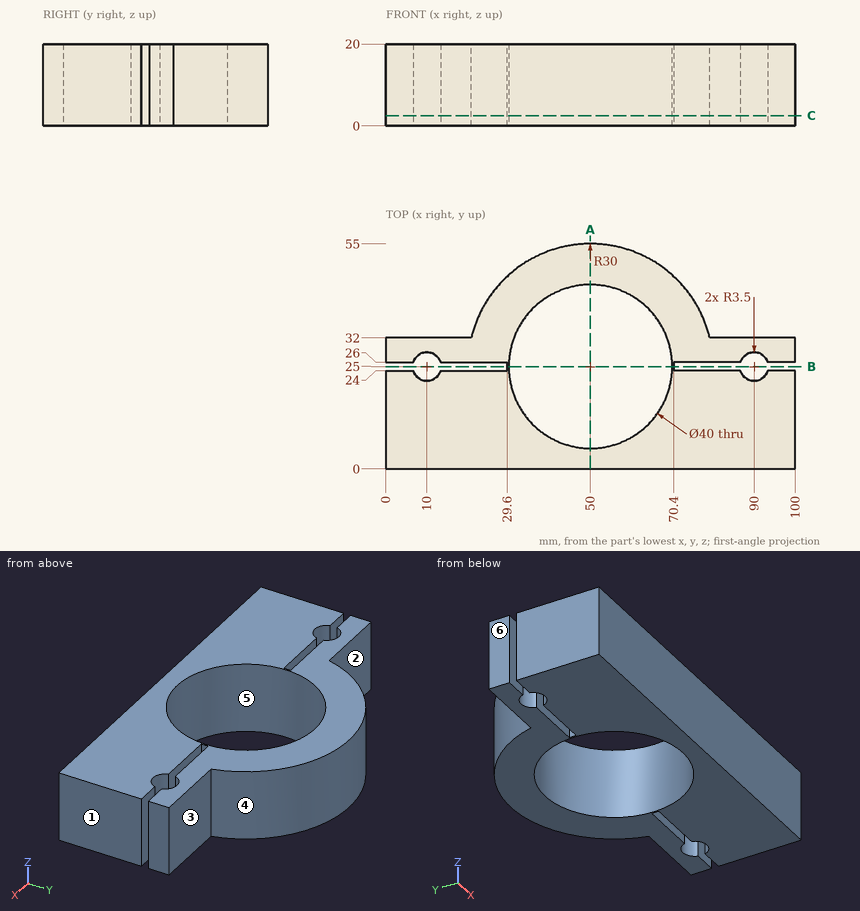
Geometry check sheet. Reference: drawing and pictorial views, mm from the part's lowest x, y, z. A direction names the side the tool comes from. Round coordinates to 2 decimals unless told otherwise and drop trailing zeros. Order: outer loops, then holes, each group sorted by start corner. A loop starts at its lowest first (then second) coordinate and runs counter-clockwise, first axis right, second up. Notation, with made-up numbers: M 62,43 L 118,43 A24 ccw 118,77 Z; hole C 75,-35.5 d10. An arc over 180 degrees is marked long. Write item = value, one per line.
Q1. Section check A-A (x = 50). Enter the section's corners in (y, z).
Answer block:
outline = M 0,0 L 5,0 L 5,20 L 0,20 Z; M 45,0 L 55,0 L 55,20 L 45,20 Z
Q2. Release check for a two-part mould opening along X. For the marked faces 4, 5 and 6 record: released by +X, released by -X, zero draft, split by the parting line, or undercut.
Answer block:
face_4 = split by the parting line
face_5 = undercut
face_6 = released by -X
Q3. Section check C-C (z = 2.5). Enter the section's corners in (x, y).
Answer block:
outline = M 0,0 L 100,0 L 100,24 L 93.35,24 A3.5 cw 86.65,24 L 70.4,24 L 70.4,26 L 86.65,26 A3.5 cw 93.35,26 L 100,26 L 100,32 L 79.17,32 A30 ccw 20.83,32 L 0,32 L 0,26 L 6.65,26 A3.5 cw 13.35,26 L 29.6,26 L 29.6,24 L 13.35,24 A3.5 cw 6.65,24 L 0,24 Z; hole C 50,25 d40
Q4. Section check B-B (y = 25). Enter the section's corners in (x, z), plus the area to 3 significant figures.
Answer block:
outline = M 29.6,0 L 30,0 L 30,20 L 29.6,20 Z; M 70,0 L 70.4,0 L 70.4,20 L 70,20 Z
area = 16.0 mm^2
Q5. Depth check by flat-ended pin: pin 1 Ø8 at (y, z) = (45, 6) entering from +X; pin 2 Ø6 at (x, z) = (85.5, 7.5) entering from +Y; pin 3 Ø2 at (y, z) = (40.5, 4.5) entering from -X. Enter the tip coordinate at first touch or a pass-through.
Answer block:
pin_1 = 75.38
pin_2 = 32
pin_3 = 23.74
Q6. Scan lines: line 1 (Y direction, x = 18.5, z = 15.25); line 2 (X direction, y = 22.5, z = 5); line 3 (X direction, y = 7, z = 1.75). Record each from-to range of solid material in increasing order.
Answer block:
line_1 = 0 to 24, 26 to 32
line_2 = 0 to 7.55, 12.45 to 30.16, 69.84 to 87.55, 92.45 to 100
line_3 = 0 to 41.28, 58.72 to 100
Q7. Set-up check for the marked faces 1, 2 and 3: record each of +Z, -Z, +X, -X, +Y, -Y from which the full face is reachable in a straight line by a thin tool's end or side.
Answer block:
face_1 = +Z, -Z, +X, +Y, -Y
face_2 = +Z, -Z, -X, +Y
face_3 = +Z, -Z, +X, +Y
